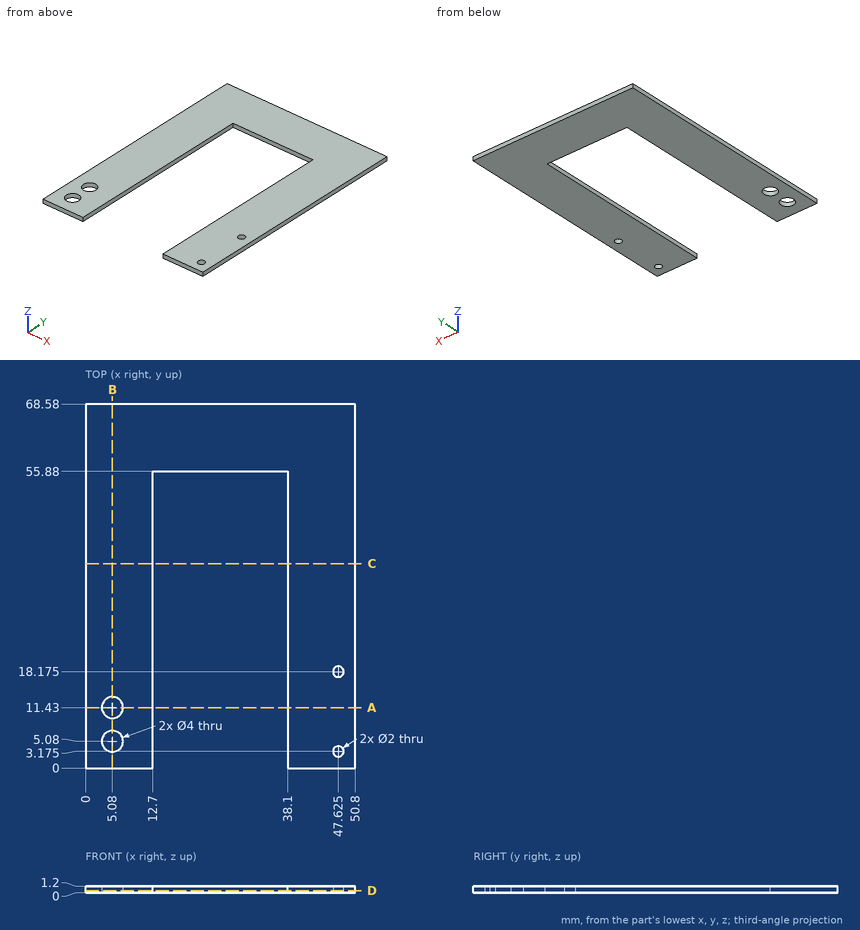
The figure shows three views and two pictorial views of one solid part (mm, origin at its lowest corner). Answer the questions. Give positions to 0.01 mm unless a question says otherwise; leave off trailing zeros. Order: outer loops, then holes, each group sorted by start corner. A loop starts at its lowest first (then second) coordinate and runs counter-clockwise, first axis right, second up. Notation, with made-up numbers: (-13, -12.5) -> (44, -12.5) arc R26 cw to (44, 16.5) -> close; hole circle Ø6 at (28, -18). An arc over 180 degrees is marked (long way). Answer as a JSON object with one key per item and string values. Group by question number.
Item 1: Consider L1, parallel to Y at x = 5.08, z = 0.65; L2, parallel to X at y = 44, z = 1.05; L3, parallel to Y at x = 32, z = 0.95. Determine where each line is inside the solid, lowest interval first. Write a range as from..to.
Item 2: The part is cut by section B-B on x = 5.08. Write down the section's boundary in (y, z).
Item 3: The part is cut by section A-A on y = 11.43. Write down the section's boundary in (x, z), and give its area (3 significant figures).
Item 4: The part is cut by section C-C on y = 38.5. Write down the section's boundary in (x, z).
Item 5: The part is cut by section D-D on z = 0.35. Write down the section's boundary in (x, y) (3 decimals), and give its area (3 significant figures).
Result set:
{
 "1": {"L1": "0..3.08, 7.08..9.43, 13.43..68.58", "L2": "0..12.7, 38.1..50.8", "L3": "55.88..68.58"},
 "2": {"outline": "(0, 0) -> (3.08, 0) -> (3.08, 1.2) -> (0, 1.2) -> close; (7.08, 0) -> (9.43, 0) -> (9.43, 1.2) -> (7.08, 1.2) -> close; (13.43, 0) -> (68.58, 0) -> (68.58, 1.2) -> (13.43, 1.2) -> close"},
 "3": {"outline": "(0, 0) -> (3.08, 0) -> (3.08, 1.2) -> (0, 1.2) -> close; (7.08, 0) -> (12.7, 0) -> (12.7, 1.2) -> (7.08, 1.2) -> close; (38.1, 0) -> (50.8, 0) -> (50.8, 1.2) -> (38.1, 1.2) -> close", "area": "25.7 mm²"},
 "4": {"outline": "(0, 0) -> (12.7, 0) -> (12.7, 1.2) -> (0, 1.2) -> close; (38.1, 0) -> (50.8, 0) -> (50.8, 1.2) -> (38.1, 1.2) -> close"},
 "5": {"outline": "(0, 0) -> (12.7, 0) -> (12.7, 55.88) -> (38.1, 55.88) -> (38.1, 0) -> (50.8, 0) -> (50.8, 68.58) -> (0, 68.58) -> close; hole circle Ø4 at (5.08, 5.08); hole circle Ø4 at (5.08, 11.43); hole circle Ø2 at (47.625, 3.175); hole circle Ø2 at (47.625, 18.175)", "area": "2,030 mm²"}
}
